```python
from build123d import *

# Parameters (mm, degrees)
SKETCH_1_R      = 10
SKETCH_1_R_2    = 1
SKETCH_1_R_3    = 3.083795415
EXTRUDE_1_DEPTH = 2
SKETCH_2_R      = 4
SKETCH_2_R_2    = 3
EXTRUDE_2_DEPTH = 2


with BuildPart() as part:
    # 草图1 → 凸台-拉伸1 (new body)
    # profile 1 of 2: a face of its own
    with BuildSketch(Plane(origin=(0, 0, 0), x_dir=(1, 0, 0), z_dir=(0, 1, 0))):
        with Locations(Location((0, 0, 0), (0, 0, 270))):
            Circle(SKETCH_1_R)
        with Locations(Location((-5, -5, 0), (0, 0, 270))):
            Circle(SKETCH_1_R_2, mode=Mode.SUBTRACT)
        with Locations(Location((5, -5, 0), (0, 0, 270))):
            Circle(SKETCH_1_R_2, mode=Mode.SUBTRACT)
        with Locations(Location((5, 5, 0), (0, 0, 270))):
            Circle(SKETCH_1_R_2, mode=Mode.SUBTRACT)
        with Locations(Location((-5, 5, 0), (0, 0, 270))):
            Circle(SKETCH_1_R_2, mode=Mode.SUBTRACT)
        Circle(SKETCH_1_R_3, mode=Mode.SUBTRACT)
    # profile 2 of 2: a face of its own
    with BuildSketch(Plane(origin=(0, 0, 0), x_dir=(1, 0, 0), z_dir=(0, 1, 0))):
        Circle(SKETCH_1_R_3)
        with Locations(Location((0, 0, 0), (0, 0, 270))):
            Circle(SKETCH_1_R_2, mode=Mode.SUBTRACT)
    extrude(amount=EXTRUDE_1_DEPTH)

    # 草图2 → 凸台-拉伸2 (add)
    with BuildSketch(Plane(origin=(0, 2, 0), x_dir=(1, 0, 0), z_dir=(0, 1, 0))):
        with Locations(Location((0, 0, 0), (0, 0, 270))):
            Circle(SKETCH_2_R)
        with Locations(Location((0, 0, 0), (0, 0, 270))):
            Circle(SKETCH_2_R_2, mode=Mode.SUBTRACT)
    extrude(amount=EXTRUDE_2_DEPTH)


solid = part.part
```
The listing builds one solid part. Answer for the finished solid, in the listing's coordinates (mm). A direction names the side the tool comes from. Round coordinates to 2 decimals unless told otherwise and drop trailing zeros. Write each loop counter-clockwise with the first axis right and the second up, starting at its lowest first coordinate (ties: lowest second). Pieces come first, ordered by that corner, then holes. Notation, with made-up numbers: (14.5, 51) -> (46.5, 51) arc R17 ccw to (46.5, 67) -> close; hole circle Ø7 at (42, 12.25). An arc over 180 degrees is marked (long way). Write item = value, one per line.
1) Straight lines are drawn through the part: line 1 along Z through (x, y) = (4.75, 1.7); line 2 along X through (y, z) = (3.25, 0); line 3 along Z through (x, y) = (-5.75, 1.8). For each, find the intervals that lie inside material, in ascending order. Write a range as [from, to].
Check values:
line_1 = [-8.8, -5.97], [-4.03, 4.03], [5.97, 8.8]
line_2 = [-4, -3], [3, 4]
line_3 = [-8.18, -5.66], [-4.34, 4.34], [5.66, 8.18]
2) For a pull along X with two mould halves and no side action, classify faces 1 (the cylindrical face through (-1, 1, 0)), 2 (the cylindrical face through (-4, 1, 5)), 3 (the flat face through (3, 4, 1)), 4 (the cylindrical face through (-9.76, 0.99, -2.17)) as released by +X, released by -X, zero draft, split by the parting line, or undercut.
Check values:
face_1 = undercut
face_2 = undercut
face_3 = zero draft
face_4 = split by the parting line
3) Section A-A on x = 5 is taken. Write down the section's boundary in (y, z), plus the area to 3 significant figures.
Check values:
outline = (0, -8.66) -> (2, -8.66) -> (2, -6) -> (0, -6) -> close; (0, -4) -> (2, -4) -> (2, 4) -> (0, 4) -> close; (0, 6) -> (2, 6) -> (2, 8.66) -> (0, 8.66) -> close
area = 26.6 mm²
4) Given pin 1 (1.6 mm diameter, centred on x = -5, z = -5, fed in from -Y); pin 2 (1.5 mm diameter, centred on x = -3.5, y = 2.5, fed in from +Z); pin 3 (2.5 mm diameter, centred on x = -5, z = 5, fed in from +Y), each flat-ended and moving along its own axis, determine where each tip first touches the part or whether it passes through.
Check values:
pin_1 = through
pin_2 = 9.56
pin_3 = 2
5) Section B-B on y = 3.35 is taken. Write down the section's boundary in (x, z), plus the area to 3 significant figures.
Check values:
outline = circle Ø8 at (0, 0); hole circle Ø6 at (0, 0)
area = 22.0 mm²
6) Section D-D on x = 0.75 is taken. Write down the section's boundary in (y, z), plus the area to 3 significant figures.
Check values:
outline = (0, -9.97) -> (2, -9.97) -> (2, -3.93) -> (4, -3.93) -> (4, -2.9) -> (2, -2.9) -> (2, -0.66) -> (0, -0.66) -> close; (0, 0.66) -> (2, 0.66) -> (2, 2.9) -> (4, 2.9) -> (4, 3.93) -> (2, 3.93) -> (2, 9.97) -> (0, 9.97) -> close
area = 41.3 mm²
7) Which of the six approach directions +Z, -Z, +X, -X, +Y, -Y give full straight-line access (tool end or side, diameter ignored) to faces 5 (the cylindrical face through (-3.905, 2.986, -0.867)), 6 (the cylindrical face through (6, 1, 5))?
Check values:
face_5 = +Y
face_6 = +Y, -Y
8) Section C-C on z = -5 is taken. Write down the section's boundary in (x, y), plus the area to 3 significant figures.
Check values:
outline = (-8.66, 0) -> (-6, 0) -> (-6, 2) -> (-8.66, 2) -> close; (-4, 0) -> (4, 0) -> (4, 2) -> (-4, 2) -> close; (6, 0) -> (8.66, 0) -> (8.66, 2) -> (6, 2) -> close
area = 26.6 mm²
